Input: part model. Units: mm. Frame: model coordinates. Coordinates: 2 decimals unless noted, no trailing zeros. Loops run counter-clockwise (first coordinate to the right, second up) from the corner with the lowest first, then second, coordinate; pieces in that order, holes last. Notation, with made-up numbers: (-3.75, 24) -> (44.25, 24) arc R24 ccw to (44.25, 39) -> close; hole circle Ø3 at (52.5, 71.25). An arc over 180 degrees is marked (long way). Answer as a JSON object with one key per item and string values.
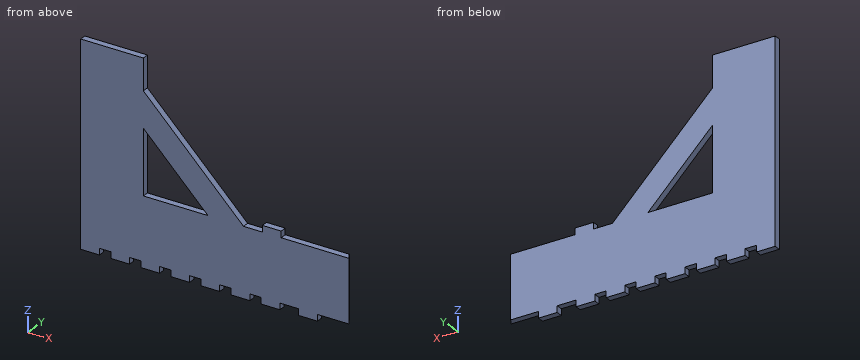
from build123d import *

# Parameters (mm, degrees)
F0_W     = 15
F0_H     = 5.08
F1_DEPTH = 5.08
F2_DEPTH = 25
F4_DEPTH = 58
F5_W     = 15
F5_H     = 5.08
F6_DEPTH = 5.08
F7_W     = 15
F7_H     = 5.08
F8_DEPTH = 5.08


# Not quite as in the source:
# - a feature names something its author has since deleted; it is built from what else it names


with BuildPart() as f1:
    # F0 (on Front) → F1 (new body)
    with BuildSketch(Plane.XZ):
        Polygon((-87.5, 0), (-32.419, 0), (-32.419, 50), (-116.5, 50), (-144.9023774395, 50), (-196.5, 50), (-196.5, 101.5976225605), (-196.5, 130), (-246.5, 130), (-246.5, 0), (-231.5, 0), (-222.5, 0), (-207.5, 0), (-198.5, 0), (-183.5, 0), (-174.5, 0), (-159.5, 0), (-150.5, 0), (-135.5, 0), (-126.5, 0), (-111.5, 0), (-102.5, 0), align=None)
        with Locations((-95, -2.54)):
            Rectangle(F0_W, F0_H)
        Polygon((-144.9023774395, 50), (-116.5, 50), (-196.5, 130), (-196.5, 101.5976225605), align=None)
        with Locations((-119, -2.54)):
            Rectangle(F0_W, F0_H)
        with Locations((-143, -2.54)):
            Rectangle(F0_W, F0_H)
        with Locations((-239, -2.54)):
            Rectangle(F0_W, F0_H)
        with Locations((-167, -2.54)):
            Rectangle(F0_W, F0_H)
        with Locations((-215, -2.54)):
            Rectangle(F0_W, F0_H)
        with Locations((-191, -2.54)):
            Rectangle(F0_W, F0_H)
    extrude(amount=F1_DEPTH)

    # F2 (add): a face of the model
    f2_faces = [f1.faces().sort_by_distance(p)[0] for p in [
        (-221.5, -2.54, 130),
    ]]
    extrude(f2_faces, amount=F2_DEPTH)

    # F3 (on face) → F4 (cut)
    with BuildSketch(Plane(origin=(0, 0, 0), x_dir=(1, 0, 0), z_dir=(0, 0, -1))):
        Polygon((-32.419, 0), (-32.419, 5.08), (-35.3519393675, 0), align=None)
    extrude(amount=-F4_DEPTH, mode=Mode.SUBTRACT)

    # F5 (on face) → F6 (join)
    with BuildSketch(Plane(origin=(0, 0, 0), x_dir=(1, 0, 0), z_dir=(0, 0, -1))):
        with Locations((-65, 2.54)):
            Rectangle(F5_W, F5_H)
    extrude(amount=F6_DEPTH)

    # F7 (on face) → F8 (join)
    with BuildSketch(Plane.XY.offset(50)):
        with Locations((-94, -2.54)):
            Rectangle(F7_W, F7_H)
    extrude(amount=F8_DEPTH)


solid = f1.part
1. Section query D-D (z = 142.5). Return loops of the section in (x, y).
Reply:
{"outline": "(-246.5, -5.08) -> (-196.5, -5.08) -> (-196.5, 0) -> (-246.5, 0) -> close"}
2. Line query: line 1 along X through (y, z) = (-2.9, 51); line 2 along X through (y, z) = (-4.85, 54); line 3 along Z through (x, y) = (-204, -0.9). Output: solid intervals per line, ascending.
Reply:
{"line 1": "x = -246.5 to -196.5, -145.9 to -117.5, -101.5 to -86.5", "line 2": "x = -246.5 to -196.5, -148.9 to -120.5, -101.5 to -86.5", "line 3": "z = 0 to 155"}
3. Section query B-B (x = -148). Return loops of the section in (y, z), plus the area to 3 significant figures.
Reply:
{"outline": "(-5.08, -5.08) -> (0, -5.08) -> (0, 50) -> (-5.08, 50) -> close; (-5.08, 53.1) -> (0, 53.1) -> (0, 81.5) -> (-5.08, 81.5) -> close", "area": "424 mm2"}
4. Section query C-C (x = -46). Return loops of the section in (y, z), plus the area to 3 significant figures.
Reply:
{"outline": "(-5.08, 0) -> (0, 0) -> (0, 50) -> (-5.08, 50) -> close", "area": "254 mm2"}
5. Pin query (flat end, axial travel): P1, Ø1, axis at x = -147, y = -2.5, coming from the +Z side; P2, Ø1.5, axis at y = -4, z = 63.5, coming from the +X side; P3, Ø1.5, axis at y = -3, z = 82.5, coming from the +X side. Return the tip coordinate at first contact, or that it passes through.
Reply:
{"P1": "stops at z = 81", "P2": "stops at x = -129.25", "P3": "stops at x = -148.25"}
6. Section query A-A (z = 83). Return loops of the section in (x, y).
Reply:
{"outline": "(-246.5, -5.08) -> (-196.5, -5.08) -> (-196.5, 0) -> (-246.5, 0) -> close; (-177.9, -5.08) -> (-149.5, -5.08) -> (-149.5, 0) -> (-177.9, 0) -> close"}
